The drawing under review shows one solid part. Ordinate dimensions are in mm from its lowest x, y, z. Round coordinates to 2 decimals unless told otherwise and drop trailing zeros. Answer as a JSON object with one key per item and string values. Group by question number.
1) To check wall thickness, follow line 1 (X direction, y = 1.5, z = 5) (1 decimal); line 2 (Z direction, x = 4.5, y = 5.5) (1 decimal); line 3 (Z direction, x = 4.75, y = 5.5) (1 decimal). State the ranges of each line that lie inside material, in increasing order.
2) Insertion check: pin 1 Ø4 at (y, z) = (2.5, 7.5) entering from +X; pin 2 Ø2 at (y, z) = (6, 5) entering from +X; pin 3 Ø4 at (y, z) = (6, 4) entering from -X; pin 4 Ø7 at (x, z) = (8.08, 7) entering from -Y. Each pin has a flat end and moves straight along its axis. Give the tip position at first contact, or say it passes through.
3) The part is to be moulded in two halves that separate along Z. For the marked faces 1, 2 and 3, say which applies: +Z half, -Z half, draft (parallel to the pull), parting line (faces both ways), or undercut.
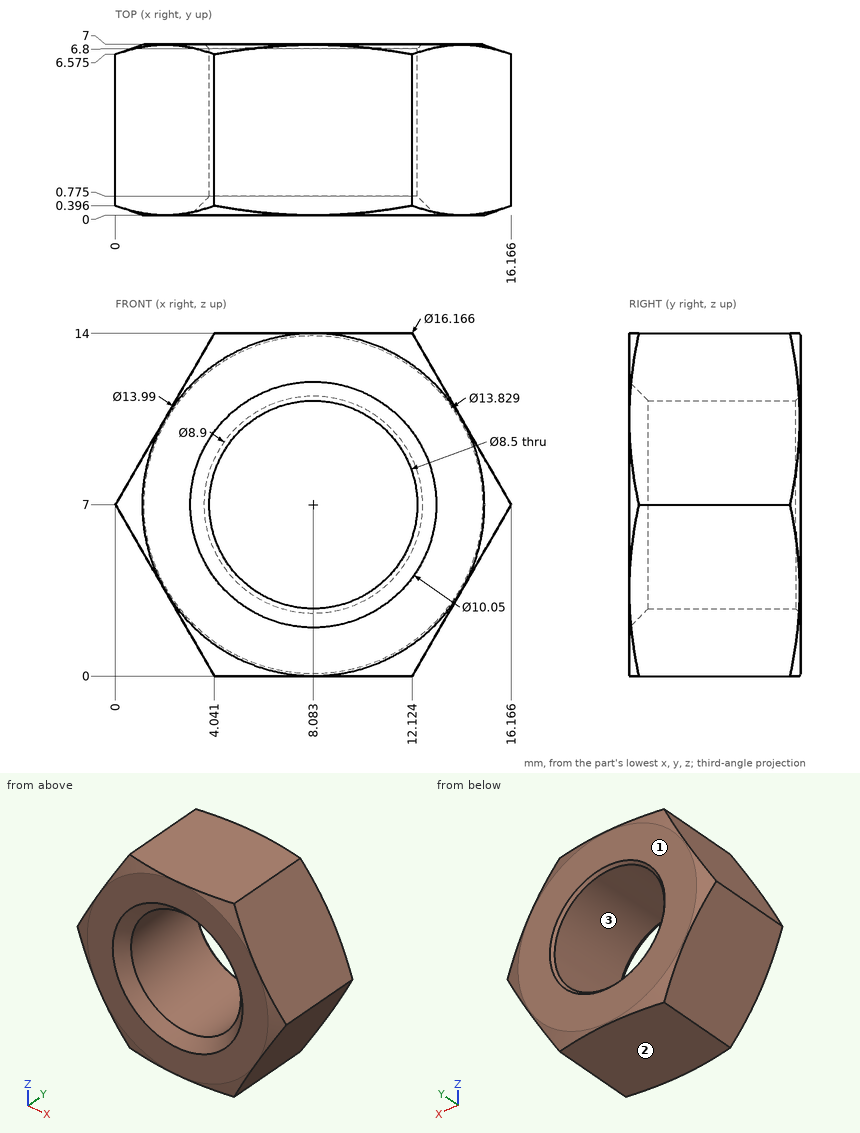
Results list:
{
 "1": {"line 1": "1.2 to 4.3, 11.8 to 15", "line 2": "0 to 4.7, 9.3 to 14", "line 3": "0 to 4.4, 9.6 to 14"},
 "2": {"pin 1": "x = 16.17", "pin 2": "x = 15.59", "pin 3": "x = 0.58", "pin 4": "through"},
 "3": {"face 1": "draft", "face 2": "-Z half", "face 3": "undercut"}
}
